Check sheet for the modelled part. Datum: model origin and axes. Units: mm. A direction names the side the tool comes from. Round coordinates to 2 decimals unless told otherwise and drop trailing zeros. Write each loop counter-clockwise with the first axis right and the second up, starting at its lowest first coordinate (ties: lowest second). Pieces come first, ordered by that corner, then holes. Notation, with made-up numbers: (39, 4) -> (92, 4) arc R26 ccw to (92, 25) -> close; hole circle Ø1 at (-3, 12). An arc over 180 degrees is marked (long way). One line per item, written item: value.
from build123d import *

# Parameters (mm, degrees)
ESQUISSE1_W              = 240
ESQUISSE1_H              = 220
ESQUISSE1_W_2            = 220
ESQUISSE1_H_2            = 200
BOSS_EXTRU_3_DEPTH       = 60
ESQUISSE1_2_W            = 240
ESQUISSE1_2_H            = 220
ESQUISSE1_2_W_2          = 220
ESQUISSE1_2_H_2          = 200
BOSS_EXTRU_4_DEPTH       = 10
ENL_V_MAT_EXTRU_17_DEPTH = 318.175030543


with BuildPart() as part:
    # Esquisse1 → Boss.-Extru.3 (new body)
    with BuildSketch(Plane.XY):
        with Locations((110, 100)):
            Rectangle(ESQUISSE1_W, ESQUISSE1_H)
        with Locations((110, 100)):
            Rectangle(ESQUISSE1_W_2, ESQUISSE1_H_2, mode=Mode.SUBTRACT)
    extrude(amount=BOSS_EXTRU_3_DEPTH)

    # Esquisse1_2 → Boss.-Extru.4 (add)
    with BuildSketch(Plane.XY):
        with Locations((110, 100)):
            Rectangle(ESQUISSE1_2_W, ESQUISSE1_2_H)
        with Locations((110, 100)):
            Rectangle(ESQUISSE1_2_W_2, ESQUISSE1_2_H_2, mode=Mode.SUBTRACT)
        with Locations((110, 100)):
            Rectangle(ESQUISSE1_2_W_2, ESQUISSE1_2_H_2)
    extrude(amount=-BOSS_EXTRU_4_DEPTH)

    # Esquisse4 → Enl_v. mat.-Extru.17 (cut, through all)
    with BuildSketch(Plane.ZY.offset(-220)):
        Polygon((365.296461205, 120), (60, 120), (50, 120), (50, 80), (60, 80), (365.296461205, 80), (975.889383614, 80), (975.889383614, 120), align=None)
    extrude(amount=-ENL_V_MAT_EXTRU_17_DEPTH, mode=Mode.SUBTRACT)


solid = part.part
Item 1: Sectioned sample at D-D (z = 55). Enter the section's corners in (x, y).
Result set:
outline: (-10, -10) -> (230, -10) -> (230, 80) -> (220, 80) -> (220, 0) -> (0, 0) -> (0, 200) -> (220, 200) -> (220, 120) -> (230, 120) -> (230, 210) -> (-10, 210) -> close
Item 2: Release check for a two-part mould opening along X. For faces 1 (the flat face through (-10, 98, 25)), 2 (the flat face through (108, 0, 30)), 3 (the flat face through (225, 120, 55)) record: pulls with the +X half, pulls with the -X half, needs draft (parallel to the pull), parting line crosses it, or undercut.
Result set:
face 1: pulls with the -X half
face 2: undercut
face 3: needs draft
Item 3: Tool access check on faces 4 (the flat face through (108, 200, 30)), 5 (the flat face through (108, 102, -10)), 6 (the flat face through (225, 100, 50)). Record the directions out of +Z, -Z, +X, -X, +Y, -Y that give a thin tool (end or side, any length) a straight path to the whole face; none if there is none.
Result set:
face 4: +Z
face 5: -Z, +X, -X, +Y, -Y
face 6: +Z, +X
Item 4: Sectioned sample at B-B (x = 161). Enter the section's corners in (y, z), then the cut area to 3 significant figures.
Result set:
outline: (-10, -10) -> (210, -10) -> (210, 60) -> (200, 60) -> (200, 0) -> (0, 0) -> (0, 60) -> (-10, 60) -> close
area: 3,400 mm^2
Item 5: Material ranges on line 1 along Y through (x, z) = (172.5, 51.5); line 2 along X through (y, z) = (31, 53.5); line 3 along Z through (x, y) = (26.5, 186.5), recorded low to high.
Result set:
line 1: -10 to 0, 200 to 210
line 2: -10 to 0, 220 to 230
line 3: -10 to 0
Item 6: Depth check by flat-ended pin: pin 1 (10 mm diameter, centred on x = 135.5, y = 168.5, fed in from +Z); pin 2 (8 mm diameter, centred on x = 223, y = 106, fed in from +Z). Enter the tip coordinate at first touch or a pass-through.
Result set:
pin 1: z = 0
pin 2: z = 50
Item 7: Sectioned sample at A-A (z = 3). Enter the section's corners in (x, y), then the cut area to 3 significant figures.
Result set:
outline: (-10, -10) -> (230, -10) -> (230, 210) -> (-10, 210) -> close; hole (0, 0) -> (220, 0) -> (220, 200) -> (0, 200) -> close
area: 8,800 mm^2
Item 8: Sectioned sample at C-C (y = 92). Enter the section's corners in (x, z), then the cut area to 3 significant figures.
Result set:
outline: (-10, -10) -> (230, -10) -> (230, 50) -> (220, 50) -> (220, 0) -> (0, 0) -> (0, 60) -> (-10, 60) -> close
area: 3,500 mm^2
